The model under review builds one solid part; all positions refer to its coordinate system, in mm. A direction names the side the tool comes from. Coordinates: 2 decimals unless noted, no trailing zeros. Write each loop counter-clockwise with the first axis right and the second up, starting at its lowest first coordinate (ties: lowest second). Pieces come first, ordered by that corner, then holes. Notation, with made-up numbers: (22.5, 20) - (71.5, 20) arc R20 ccw to (71.5, 55) - close; hole circle Ø7 at (84.25, -18). An arc over 180 degrees is marked (long way). Put each result on its own line as item: value.
from build123d import *

# Parameters (mm, degrees)
SKETCH1_W           = 115
SKETCH1_H           = 65
BOSS_EXTRUDE1_DEPTH = 30
BOSS_EXTRUDE2_DEPTH = 4
SKETCH4_R           = 5
BOSS_EXTRUDE3_DEPTH = 30
FILLET1_R           = 8


with BuildPart() as part:
    # Sketch1 → Boss-Extrude1 (new body)
    with BuildSketch(Plane(origin=(0, 0, 0), x_dir=(1, 0, 0), z_dir=(0, 1, 0))):
        Rectangle(SKETCH1_W, SKETCH1_H)
    extrude(amount=BOSS_EXTRUDE1_DEPTH)

    # Sketch3 → Boss-Extrude2 (add)
    with BuildSketch(Plane.XZ):
        with BuildLine():
            Line((-70.5, 10), (70.5, 10))
            Line((70.5, 10), (70.5, 2))
            Line((70.5, 2), (63.5, 2))
            ThreePointArc((63.5, 2), (61.5, 0), (63.5, -2))
            Line((63.5, -2), (70.5, -2))
            Line((70.5, -2), (70.5, -10))
            Line((70.5, -10), (-70.5, -10))
            Line((-70.5, -10), (-70.5, -2))
            Line((-70.5, -2), (-63.5, -2))
            ThreePointArc((-63.5, -2), (-61.5, 0), (-63.5, 2))
            Line((-63.5, 2), (-70.5, 2))
            Line((-70.5, 2), (-70.5, 10))
        make_face()
    extrude(amount=-BOSS_EXTRUDE2_DEPTH)

    # Sketch4 → Boss-Extrude3 (add)
    with BuildSketch(Plane(origin=(57.5, 0, 0), x_dir=(0, 0, -1), z_dir=(1, 0, 0))):
        with Locations(Location((14.5, 18, 0), (0, 0, 180))):
            Circle(SKETCH4_R)
    extrude(amount=BOSS_EXTRUDE3_DEPTH)

    # Fillet1
    fillet1_edges = [part.edges().sort_by_distance(p)[0] for p in [
        (-57.5, 15, -32.5),
        (57.5, 15, -32.5),
        (57.5, 15, 32.5),
        (-57.5, 15, 32.5),
    ]]
    fillet(fillet1_edges, radius=FILLET1_R)


solid = part.part
1. To check wall thickness, follow probe 1 along X at (y, z) = (28, 10.5); probe 2 along X at (y, z) = (1.5, 8); probe 3 along Y at (x, z) = (58.5, 3.5). State the ranges of each line that lie inside material, in increasing order.
Determined:
probe 1: x = -57.5 to 57.5
probe 2: x = -70.5 to 70.5
probe 3: y = 0 to 4
2. Consider section C-C on x = -55.5. State the section outline as (y, z) points, plus the area to 3 significant figures.
Determined:
outline: (0, -29.79) - (30, -29.79) - (30, 29.79) - (0, 29.79) - close
area: 1,790 mm^2
3. For pin 1 Ø4.5 at (x, y) = (-67, 1) entering from +Z; pin 2 Ø1 at (x, y) = (-50.5, 16) entering from -Z; pin 3 Ø10.5 at (x, z) = (65, 3.5) entering from +Y, all flat-tipped, find the tip position at first contact; note any pin that passes through.
Determined:
pin 1: stops at z = 10
pin 2: stops at z = -32.48
pin 3: stops at y = 4
4. Consider section B-B on y = 18. State the section outline as (x, z) points.
Determined:
outline: (-57.5, -24.5) arc R8 ccw to (-49.5, -32.5) - (49.5, -32.5) arc R8 ccw to (57.5, -24.5) - (57.5, -19.5) - (87.5, -19.5) - (87.5, -9.5) - (57.5, -9.5) - (57.5, 24.5) arc R8 ccw to (49.5, 32.5) - (-49.5, 32.5) arc R8 ccw to (-57.5, 24.5) - close
5. Consider section D-D on z = -22. State the section outline as (x, y) points, plus the area to 3 significant figures.
Determined:
outline: (-57.5, 0) - (57.5, 0) - (57.5, 30) - (-57.5, 30) - close
area: 3,450 mm^2
6. Machinability: for faces 1 (the flat face through (-63.9, 4, 2.4)), 2 (the flat face through (64, 2, 10)), 3 (the flat face through (-64, 2, -10)), 4 (the flat face through (-67, 2, 2)), which of the approach directions +Z, -Z, +X, -X, +Y, -Y give a long, thin tool a straight path to every point of the face, cutting with its end or side? Answer none if there is none.
Determined:
face 1: +Z, -Z, -X, +Y
face 2: +Z, +X, +Y, -Y
face 3: -Z, -X, +Y, -Y
face 4: -X, +Y, -Y
7. The part is to be moulded in two halves that separate along Z. For faces 5 (the flat face through (67, 2, -2)), 6 (the flat face through (70.5, 2, -6)), 7 (the cylindrical face through (-55.219, 15.21, 30.094)), say which applies: +Z half, -Z half, draft (parallel to the pull), parting line (faces both ways), or undercut.
Determined:
face 5: undercut
face 6: draft
face 7: +Z half
8. Consider section A-A on z = -14.5. State the section outline as (x, y) points.
Determined:
outline: (-57.5, 0) - (57.5, 0) - (57.5, 13) - (87.5, 13) - (87.5, 23) - (57.5, 23) - (57.5, 30) - (-57.5, 30) - close
